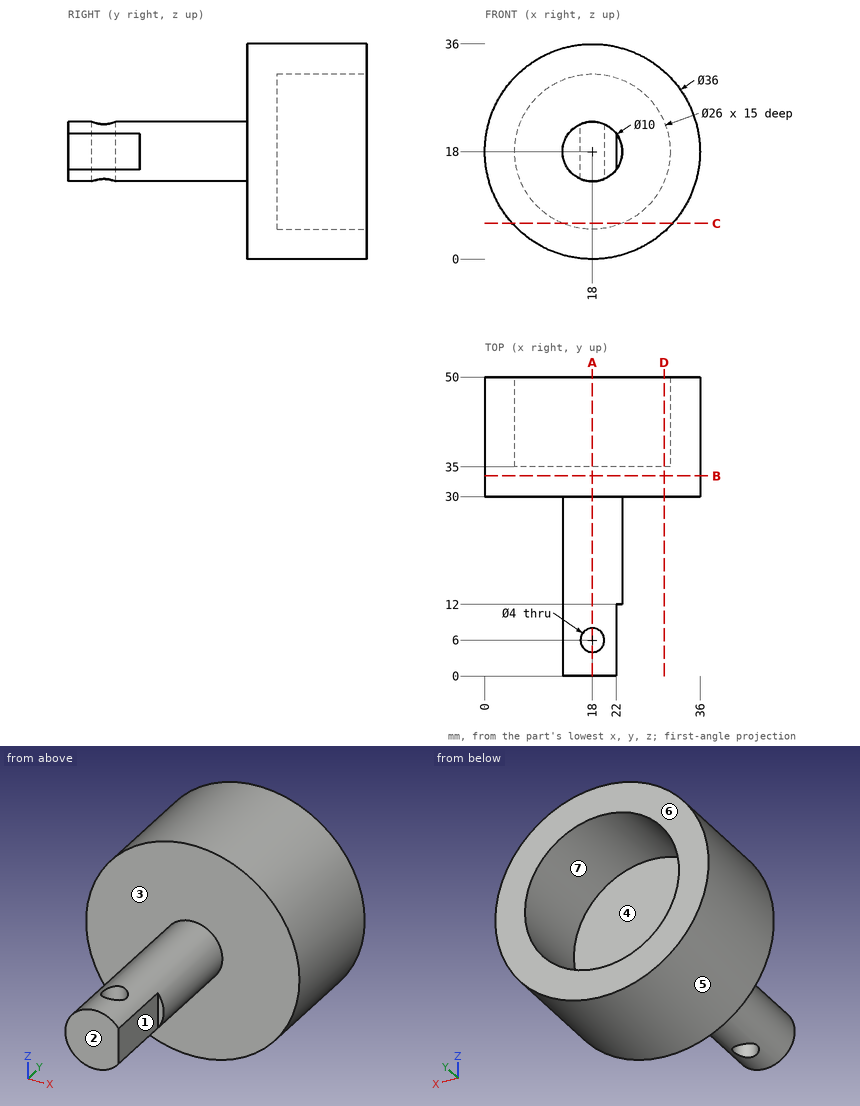
Input: dimensioned drawing with shaded views. Units: mm. Origin: part minimum x, y, z. A direction names the side the tool comes from. Coordinates: 2 decimals unless noted, no trailing zeros. Order: outer loops, then holes, each group sorted by start corner. A loop starts at its lowest first (then second) coordinate and runs counter-clockwise, first axis right, second up. Notation, with made-up numbers: M -22.75,45 L -0.75,45 A27 ccw -0.75,79 Z; hole C 82,10 d6. An arc over 180 degrees is marked long. Answer as CSV lines item,"result".
Q1. First-contact query: P1, Ø3, axis at y = 5.5, z = 18, coming from the +X side; P2, Ø3, axis at y = 16, z = 19.5, coming from the -X side; P3, Ø4, axis at x = 28, z = 18.5, coming from the +Y side. Flat tips, straight axial feed; report the tip coordinate or a pass-through.
Answers:
P1,"stops at x = 22"
P2,"stops at x = 13"
P3,"stops at y = 35"
Q2. Line query: probe 1 along Y at (x, z) = (18, 20); probe 2 along Z at (x, y) = (18, 40.5). Output: solid intervals per line, ascending. Write a range as [from, to].
Answers:
probe 1,"y = [0, 4], [8, 35]"
probe 2,"z = [0, 5], [31, 36]"
Q3. Section B-B on y = 33.5. Return the cut outline in (x, z), and give its area (3 significant figures).
Answers:
outline,"C 18,18 d36"
area,"1,020 mm^2"
Q4. Set-up query: the marked faces 1, 2, 3 and 4. Return all of +Z, -Z, +X, -X, +Y, -Y with unobstructed straight access to the full face (end or side cutting, diameter ignored); none if empty.
Answers:
face 1,"+Z, -Z, +X, -Y"
face 2,"+Z, -Z, +X, -X, -Y"
face 3,"-Y"
face 4,"+Y"
Q5. Section C-C on z = 6. Return the cut outline in (x, y), and give its area (3 significant figures).
Answers:
outline,"M 4.58,30 L 31.42,30 L 31.42,50 L 23,50 L 23,35 L 13,35 L 13,50 L 4.58,50 Z"
area,"387 mm^2"
Q6. Draft query along X for the marked faces 5, 6 and 7. Return one class per face: pulls with the +X half, pulls with the -X half, needs draft (parallel to the pull), parting line crosses it, or undercut.
Answers:
face 5,"parting line crosses it"
face 6,"needs draft"
face 7,"undercut"
Q7. Section A-A on x = 18. Return the cut outline in (y, z).
Answers:
outline,"M 0,13 L 4,13 L 4,23 L 0,23 Z; M 8,13 L 30,13 L 30,0 L 50,0 L 50,5 L 35,5 L 35,31 L 50,31 L 50,36 L 30,36 L 30,23 L 8,23 Z"
Q8. Section D-D on x = 30. Return the cut outline in (y, z), and give its area (3 significant figures).
Answers:
outline,"M 30,4.58 L 50,4.58 L 50,13 L 35,13 L 35,23 L 50,23 L 50,31.42 L 30,31.42 Z"
area,"387 mm^2"
